Autodesk Inventor part; units mm, degrees
ref_plane "YZ Plane" through (0, 0, 0) normal (1, 0, 0) x (0, 1, 0)
ref_plane "XZ Plane" through (0, 0, 0) normal (0, 1, 0) x (-1, 0, 0)
ref_plane "XY Plane" through (0, 0, 0) normal (0, 0, 1) x (1, 0, 0)
sketch "Sketch1" plane through (0, 0, 0) normal (0, 0, 1) x (1, 0, 0)
  circle A0 centre (0, 0) radius 40
  dimension "d1" = 80
extrude "Extrusion1" add sketch "Sketch1" along normal blind 800
sketch "Sketch2" plane through (0, 0, 800) normal (0, 0, 1) x (1, 0, 0)
  circle A0 centre (0, 0) radius 42
  dimension "d4" = 84
extrude "Extrusion2" add sketch "Sketch2" along normal blind 3
sketch "Sketch3" plane through (0, 0, 0) normal (0, 0, -1) x (-1, 0, 0)
  circle A0 centre (0, 0) radius 42
  dimension "d9" = 84
extrude "Extrusion3" add sketch "Sketch3" along normal blind 3
sketch "Sketch4" plane through (0, 0, 803) normal (0, 0, 1) x (1, 0, 0)
  circle A0 centre (0, 0) radius 10
  dimension "d10" = 20
extrude "Extrusion4" add sketch "Sketch4" along normal blind 8
sketch "Sketch5" plane through (0, 0, -3) normal (0, 0, -1) x (-1, 0, 0)
  circle A0 centre (0, 0) radius 10
  circle A1 centre (0, 0) radius 10
extrude "Extrusion5" add sketch "Sketch5" along normal blind 8
sketch "Sketch6" plane through (0, 0, -11) normal (0, 0, -1) x (-1, 0, 0)
  circle A0 centre (0, 0) radius 50
  dimension "d15" = 100
extrude "Extrusion6" add sketch "Sketch6" along normal blind 5
sketch "Sketch7" plane through (0, 0, 811) normal (0, 0, 1) x (1, 0, 0)
  circle A0 centre (0, 0) radius 50
extrude "Extrusion7" add sketch "Sketch7" along normal blind 5
properties part number "TrucBangTai"
Model file for the job. Use its own axes, mm. A direction names the side the tool comes from. Coordinates: 2 decimals unless noted, no trailing zeros. Order: outer loops, then holes, each group sorted by start corner. A loop starts at its lowest first (then second) coordinate and runs counter-clockwise, first axis right, second up. Notation, with made-up numbers: (40, 3.5) -> (79, 3.5) arc R18 cw to (79, 33.5) -> close; hole circle Ø9 at (43.25, -21.75). An arc over 180 degrees is marked (long way). Return JSON: item names as keys, results as strings. Group by question number.
Item 1: Wall check: line 1 along Z through (x, y) = (-12, -28); line 2 along Z through (x, y) = (-45, -19); line 3 along Y through (x, z) = (2, 215). Give the ranges that are in metal, low to high. Write a range as [from, to].
Item 2: Saw through at A-A on x = 32. Write the cut outline in (y, z), then the cut area to 3 significant figures.
Item 3: Tool access for faces 1 (the flat face through (37.1, -15.4, 800)), 2 (the flat face through (-1, 1, 816)): list every direction of +Z, -Z, +X, -X, +Y, -Y with a clear straight run to the whole face (end or side of a thin tool).
Item 4: Flat gauge pins, fed straight in: P1, Ø4, axis at y = -37, z = 138.5, coming from the +X side; P2, Ø5, axis at x = 31, z = 606.5, coming from the +Y side; P3, Ø1.5, axis at x = -3, z = 482, coming from the -Y side. Where does each tip first touch, or does it go through?
Item 5: Saw through at B-B on y = 0. Write the cut outline in (x, z).
Values found:
{
 "1": {"line 1": "z = [-16, -11], [-3, 803], [811, 816]", "line 2": "z = [-16, -11], [811, 816]", "line 3": "y = [-39.95, 39.95]"},
 "2": {"outline": "(-38.42, -16) -> (38.42, -16) -> (38.42, -11) -> (-38.42, -11) -> close; (-38.42, 811) -> (38.42, 811) -> (38.42, 816) -> (-38.42, 816) -> close; (-27.2, -3) -> (27.2, -3) -> (27.2, 0) -> (24, 0) -> (24, 800) -> (27.2, 800) -> (27.2, 803) -> (-27.2, 803) -> (-27.2, 800) -> (-24, 800) -> (-24, 0) -> (-27.2, 0) -> close", "area": "39,500 mm2"},
 "3": {"face 1": "none", "face 2": "+Z, +X, -X, +Y, -Y"},
 "4": {"P1": "stops at x = 19.36", "P2": "stops at y = 28.07", "P3": "stops at y = -39.94"},
 "5": {"outline": "(-50, -16) -> (50, -16) -> (50, -11) -> (10, -11) -> (10, -3) -> (42, -3) -> (42, 0) -> (40, 0) -> (40, 800) -> (42, 800) -> (42, 803) -> (10, 803) -> (10, 811) -> (50, 811) -> (50, 816) -> (-50, 816) -> (-50, 811) -> (-10, 811) -> (-10, 803) -> (-42, 803) -> (-42, 800) -> (-40, 800) -> (-40, 0) -> (-42, 0) -> (-42, -3) -> (-10, -3) -> (-10, -11) -> (-50, -11) -> close"}
}
